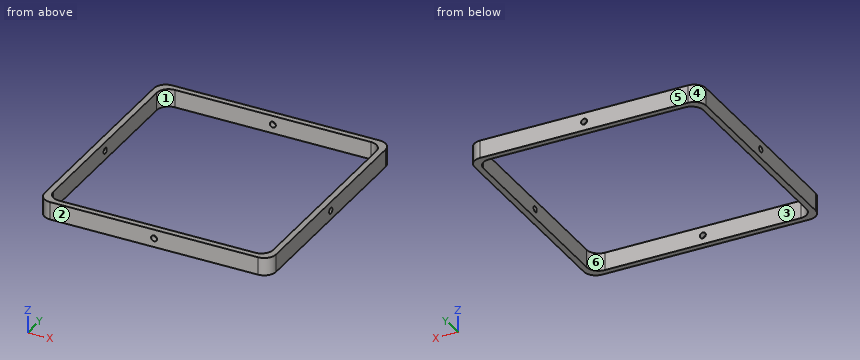
```python
from build123d import *

# Parameters (mm, degrees)
F0_W     = 194.99999
F0_H     = 194.99999
F0_W_2   = 185
F0_H_2   = 185
F1_DEPTH = 15
F2_R     = 10
F3_R     = 2.5
F4_DEPTH = 195.00099
F5_R     = 2.5
F6_DEPTH = 195.00099


with BuildPart() as f1:
    # F0 (on Top) → F1 (new body)
    with BuildSketch(Plane.XY):
        Rectangle(F0_W, F0_H)
        Rectangle(F0_W_2, F0_H_2, mode=Mode.SUBTRACT)
    extrude(amount=F1_DEPTH)

    # F2
    f2_edges = [f1.edges().sort_by_distance(p)[0] for p in [
        (-97.499995, -97.499995, 7.5),
        (97.499995, -97.499995, 7.5),
        (92.5, 92.5, 7.5),
        (-97.499995, 97.499995, 7.5),
        (97.499995, 97.499995, 7.5),
        (92.5, -92.5, 7.5),
        (-92.5, -92.5, 7.5),
        (-92.5, 92.5, 7.5),
    ]]
    fillet(f2_edges, radius=F2_R)

    # F3 (on face) → F4 (cut, through all)
    with BuildSketch(Plane.YZ.offset(97.499995)):
        with Locations((0, 7.5)):
            Circle(F3_R)
    extrude(amount=-F4_DEPTH, mode=Mode.SUBTRACT)

    # F5 (on face) → F6 (cut, through all)
    with BuildSketch(Plane.XZ.offset(97.499995)):
        with Locations((0, 7.5)):
            Circle(F5_R)
    extrude(amount=-F6_DEPTH, mode=Mode.SUBTRACT)


solid = f1.part
```
Part model, mm, in its own coordinate system. Face numbers are marked on the shaded views. A direction names the side the tool comes from. Give positions to 0.01 mm unless a question says otherwise; leave off trailing zeros. Loops run counter-clockwise (first coordinate to the right, second up) from the corner with the lowest first, then second, coordinate; pieces in that order, holes last. Notation, with made-up numbers: M -22,4 L 11,4 A22 cw 11,28 Z; hole C 12,38 d8. An arc over 180 degrees is marked long. Return JSON: item names as keys, results as strings.
1) Drill centre lines: line 1 (Y direction, x = 53, z = 14); line 2 (Z direction, x = -95, y = 0). Where is each one in solid material? Low to high.
Calculated:
{"line 1": "y = -97.5 to -92.5, 92.5 to 97.5", "line 2": "z = 0 to 5, 10 to 15"}
2) 3-axis set-ups, long thin cutter, end or side, ignore diameter. For the marked faces 1 and 2: which of +Z, -Z, +X, -X, +Y, -Y reach the whole face in a straight line?
Calculated:
{"face 1": "+Z, -Z", "face 2": "+Z, -Z, +X, -X, -Y"}
3) Flat gauge pins, fed straight in: pin 1 Ø8 at (x, z) = (0, 7.5) entering from -Y; pin 2 Ø3 at (y, z) = (0.5, 7) entering from +X. Where does each tip first touch, or does it go through?
Calculated:
{"pin 1": "stops at y = -97.5", "pin 2": "passes through"}
4) Pull direction X, two halves, no side cores. Call the marked faces 3, 4, 5 and 6: released by +X, released by -X, zero draft, split by the parting line, or undercut.
Calculated:
{"face 3": "undercut", "face 4": "released by -X", "face 5": "zero draft", "face 6": "undercut"}
5) Saw through at A-A, the plane y = 0. List the corners of the cut face in (x, z).
Calculated:
{"outline": "M -97.5,0 L -92.5,0 L -92.5,5 L -97.5,5 Z; M -97.5,10 L -92.5,10 L -92.5,15 L -97.5,15 Z; M 92.5,0 L 97.5,0 L 97.5,5 L 92.5,5 Z; M 92.5,10 L 97.5,10 L 97.5,15 L 92.5,15 Z"}
6) Saw through at C-C, the plane z = 7.5. Count the separate pieces of the cut face and the enclosed holes in it, then the cut area to 3 significant figures.
Calculated:
{"separate pieces": "4", "enclosed holes": "0", "area": "3,700 mm2"}
7) Saw through at B-B, the plane x = -25. List the corners of the cut face in (y, z).
Calculated:
{"outline": "M -97.5,0 L -92.5,0 L -92.5,15 L -97.5,15 Z; M 92.5,0 L 97.5,0 L 97.5,15 L 92.5,15 Z"}
